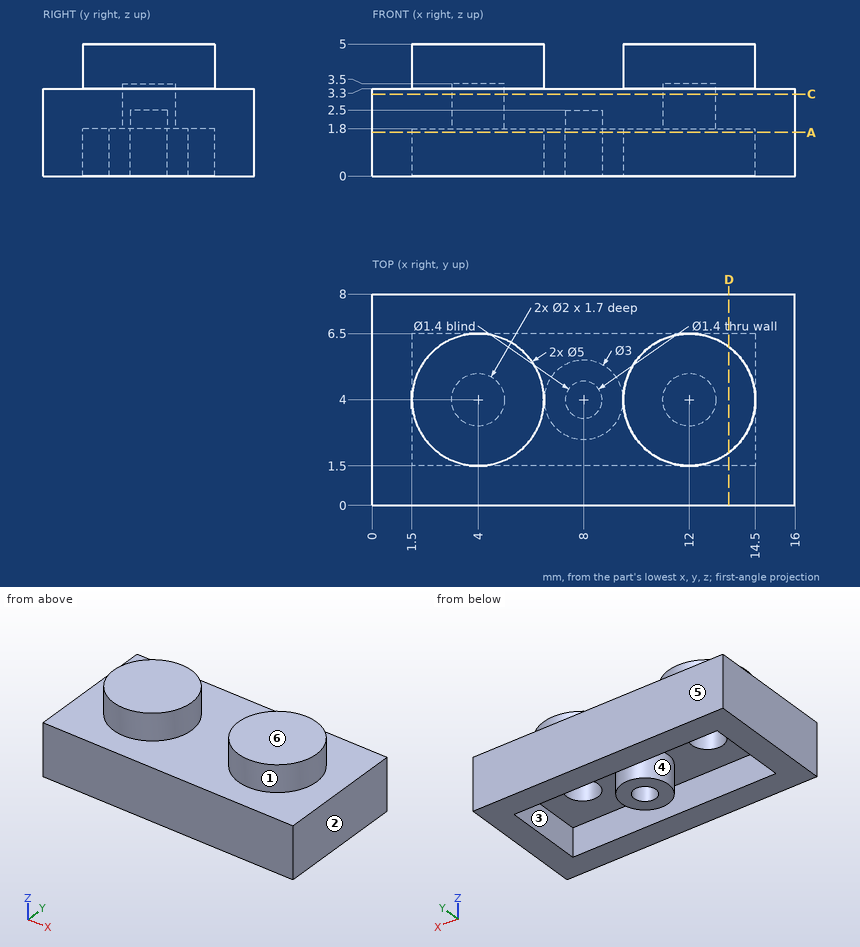
Check sheet for the drawn part. Datum: minimum x, y, z corner. Units: mm. A direction names the side the tool comes from. Round coordinates to 2 decimals unless told otherwise and drop trailing zeros. Write each loop counter-clockwise with the first axis right and the second up, starting at its lowest first coordinate (ties: lowest second). Pieces come first, ordered by that corner, then holes. Notation, with made-up numbers: (56, 77.25) -> (74, 77.25) arc R38 cw to (74, 115.25) -> close; hole circle Ø5 at (-34.75, 6). An arc over 180 degrees is marked (long way). Write each question's results on one line, items separated by ' | '. Start each with the question number.
1. Set-up check for the marked faces 1, 2 and 3: record each of +Z, -Z, +X, -X, +Y, -Y from which the full face is reachable in a straight line by a thin tool's end or side.
2. Cross-section at D-D (x = 13.5). Enter the section's corners in (y, z), then the cut area to 3 significant figures.
3. Cross-section at A-A (z = 1.65). Enter the section's corners in (x, y), then the cut area to 3 significant figures.
4. Depth check by flat-ended pin: P1, Ø2, axis at x = 4, y = 4.5, coming from the -Z side; P2, Ø1.6, axis at x = 8, y = 4, coming from the +Z side. Enter the tip coordinate at first touch or a pass-through.
5. Cross-section at C-C (z = 3.1). Enter the section's corners in (x, y).
6. Material ranges on probe 1 along Y at (x, z) = (8, 1.15); probe 2 along X at (y, z) = (4, 2.05); probe 3 along X at (y, z) = (4, 2.8), recorded low to high. Write a range as from..to.
7. Draft check along Y on the marked faces 4, 5 and 6. Enter one of: +Y half, -Y half, draft (parallel to the pull), parting line (faces both ways), or undercut.
Solutions:
1) face 1: +Z | face 2: +Z, -Z, +X, +Y, -Y | face 3: -Z
2) outline: (0, 0) -> (1.5, 0) -> (1.5, 1.8) -> (6.5, 1.8) -> (6.5, 0) -> (8, 0) -> (8, 3.3) -> (6, 3.3) -> (6, 5) -> (2, 5) -> (2, 3.3) -> (0, 3.3) -> close | area: 24.2 mm2
3) outline: (0, 0) -> (16, 0) -> (16, 8) -> (0, 8) -> close; circle Ø3 at (8, 4); hole (1.5, 1.5) -> (14.5, 1.5) -> (14.5, 6.5) -> (1.5, 6.5) -> close; hole circle Ø1.4 at (8, 4) | area: 68.5 mm2
4) P1: stops at z = 1.8 | P2: stops at z = 3.3
5) outline: (0, 0) -> (16, 0) -> (16, 8) -> (0, 8) -> close; hole circle Ø2 at (4, 4); hole circle Ø2 at (12, 4)
6) probe 1: y = 0..1.5, 2.5..3.3, 4.7..5.5, 6.5..8 | probe 2: x = 0..3, 5..7.3, 8.7..11, 13..16 | probe 3: x = 0..3, 5..11, 13..16
7) face 4: undercut | face 5: +Y half | face 6: draft
